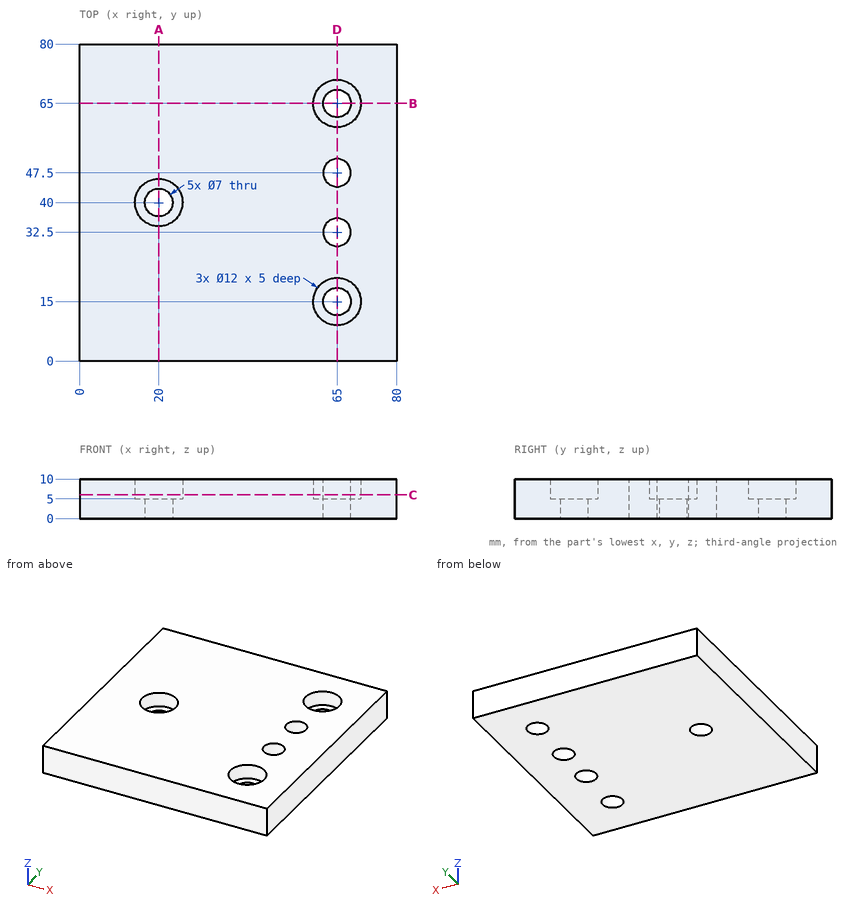
Print and shaded views of the part. All mm, measured from the part's lowest x, y and z. Round coordinates to 2 decimals unless told otherwise and drop trailing zeros. Write each loop counter-clockwise with the first axis right and the second up, starting at its lowest first coordinate (ties: lowest second). Pieces come first, ordered by that corner, then holes.
(1) Drop a flat-ended pin along its axis: P1, Ø3.5, axis at x = 65, y = 63, coming from the +Z side. Give the stop position or say it passes through.
(2) Slice it at A-A, the plane x = 20. Write the cut outline in (y, z), and give its area (3 significant figures).
(3) Slice it at C-C, the plane z = 6. Write the cut outline in (x, y), and give its area (3 significant figures).
(4) Slice it at D-D, the plane x = 65. Write the cut outline in (y, z), and give its area (3 significant figures).
(5) Probe line 1 along Y through (x, z) = (65, 6.75); line 2 along X through (y, z) = (15, 7.65); line 3 along X through (y, z) = (45, 5.25). List the from-to ranges inside material, lowest first.
(6) Slice it at B-B, the plane y = 65. Write the cut outline in (x, z), and give its area (3 significant figures).
From the geometry:
1. P1: stops at z = 5
2. outline: (0, 0) - (36.5, 0) - (36.5, 5) - (34, 5) - (34, 10) - (0, 10) - close; (43.5, 0) - (80, 0) - (80, 10) - (46, 10) - (46, 5) - (43.5, 5) - close
2. area: 705 mm2
3. outline: (0, 0) - (80, 0) - (80, 80) - (0, 80) - close; hole circle Ø12 at (20, 40); hole circle Ø12 at (65, 15); hole circle Ø12 at (65, 65); hole circle Ø7 at (65, 32.5); hole circle Ø7 at (65, 47.5)
3. area: 5,980 mm2
4. outline: (0, 0) - (11.5, 0) - (11.5, 5) - (9, 5) - (9, 10) - (0, 10) - close; (18.5, 0) - (29, 0) - (29, 10) - (21, 10) - (21, 5) - (18.5, 5) - close; (36, 0) - (44, 0) - (44, 10) - (36, 10) - close; (51, 0) - (61.5, 0) - (61.5, 5) - (59, 5) - (59, 10) - (51, 10) - close; (68.5, 0) - (80, 0) - (80, 10) - (71, 10) - (71, 5) - (68.5, 5) - close
4. area: 470 mm2
5. line 1: y = 0 to 9, 21 to 29, 36 to 44, 51 to 59, 71 to 80
5. line 2: x = 0 to 59, 71 to 80
5. line 3: x = 0 to 16.68, 23.32 to 62.55, 67.45 to 80
6. outline: (0, 0) - (61.5, 0) - (61.5, 5) - (59, 5) - (59, 10) - (0, 10) - close; (68.5, 0) - (80, 0) - (80, 10) - (71, 10) - (71, 5) - (68.5, 5) - close
6. area: 705 mm2
